```python
from build123d import *

# Parameters (mm, degrees)
SKETCH_W     = 79.03
SKETCH_H     = 8.7
PAD_DEPTH    = 1.6
SKETCH001_R  = 1.5
POCKET_DEPTH = 1.601
FILLET_R     = 5
FILLET001_R  = 1
CHAMFER_SIZE = 1.599


with BuildPart() as part:
    # Sketch → Pad (new body)
    with BuildSketch(Plane.XY):
        with Locations((0, 4.35)):
            Rectangle(SKETCH_W, SKETCH_H)
    extrude(amount=PAD_DEPTH)

    # Sketch001 (on Face6 of Pad) → Pocket (cut, through all)
    with BuildSketch(Plane.XY.offset(1.6)):
        with Locations((-33.34, 3.5)):
            Circle(SKETCH001_R)
        with Locations((33.34, 3.5)):
            Circle(SKETCH001_R)
    extrude(amount=-POCKET_DEPTH, mode=Mode.SUBTRACT)

    # Fillet
    fillet_edges = [part.edges().sort_by_distance(p)[0] for p in [
        (39.515, 8.7, 0.8),
        (-39.515, 8.7, 0.8),
    ]]
    fillet(fillet_edges, radius=FILLET_R)

    # Fillet001
    fillet001_edges = [part.edges().sort_by_distance(p)[0] for p in [
        (-38.050534, 7.235534, 1.6),
    ]]
    fillet(fillet001_edges, radius=FILLET001_R)

    # Chamfer
    chamfer_edges = [part.edges().sort_by_distance(p)[0] for p in [
        (31.84, 3.5, 1.6),
        (-34.84, 3.5, 1.6),
    ]]
    chamfer(chamfer_edges, length=CHAMFER_SIZE)


solid = part.part
```
Model file for the job. Use its own axes, mm. Coordinates: 2 decimals unless noted, no trailing zeros. Loops run counter-clockwise (first coordinate to the right, second up) from the corner with the lowest first, then second, coordinate; pieces in that order, holes last. Notation, with made-up numbers: (-35, -32) - (-18, -32) arc R12 cw to (-18, -17) - close; hole circle Ø5 at (-27, 37). An arc over 180 degrees is marked (long way). Answer as a JSON object with one key per item and string values. Group by question number.
(1) Flat gauge pin, fed straight in: pin 1 (1.8 mm diameter, centred on x = 33.34, y = 3.5, fed in from +Z). Where does the tip first touch, or does it go through?
(2) Probe line 1 along X through (y, z) = (3.5, 0.05) (3 decimals); line 2 along X through (y, z) = (4.5, 1); line 3 along Y through (x, z) = (-33.34, 0.05). List the from-to ranges inside material, lowest first.
(3) Cut at B-B (x = 13). Give the cut face in (y, z), then the cut area to 3 significant figures.
Geometry says:
{
 "1": {"pin 1": "passes through"},
 "2": {"line 1": "x = -39.515 to -34.889, -31.791 to 31.791, 34.889 to 39.515", "line 2": "x = -39.37 to -35.63, -31.05 to 31.05, 35.63 to 39.37", "line 3": "y = 0 to 1.95, 5.05 to 8.7"},
 "3": {"outline": "(0, 0) - (8.7, 0) - (8.7, 0.6) arc R1 ccw to (7.7, 1.6) - (0, 1.6) - close", "area": "13.7 mm^2"}
}
